from build123d import *
from build123d.topology import SkipClean

# Parameters (mm, degrees)
SKETCH_1_R          = 1.5
EXTRUDE_1_DEPTH     = 15
SKETCH_2_R          = 5
SKETCH_2_R_2        = 1.5
EXTRUDE_2_DEPTH     = 4
FILLET_1_R          = 1
SKETCH_3_R          = 1.5
CUT_EXTRUDE_1_DEPTH = 19
SKETCH_4_R          = 3.4
CUT_EXTRUDE_3_DEPTH = 19


with BuildPart() as part:
    # 草图1 → 凸台-拉伸1 (new body)
    with BuildSketch(Plane.XY):
        with BuildLine():
            Line((0, 0), (50, 0))
            Line((50, 0), (50, 8))
            Line((50, 8), (27.250210303, 19.465036796))
            ThreePointArc((27.250210303, 19.465036796), (25, 20), (22.749789697, 19.465036796))
            Line((22.749789697, 19.465036796), (0, 8))
            Line((0, 8), (0, 0))
        make_face()
        with Locations((25, 15)):
            Circle(SKETCH_1_R, mode=Mode.SUBTRACT)
    extrude(amount=EXTRUDE_1_DEPTH)

    # 草图2 → 凸台-拉伸2 (add)
    with BuildSketch(Plane.XY.offset(15)):
        with Locations(Location((25, 15, 0), (0, 0, 116.746382546))):
            Circle(SKETCH_2_R)
        with Locations((25, 15)):
            Circle(SKETCH_2_R_2, mode=Mode.SUBTRACT)
    extrude(amount=EXTRUDE_2_DEPTH)

    # 圆角1
    fillet_1_edges = [part.edges().sort_by_distance(p)[0] for p in [
        (27.250210303, 10.534963204, 19),
    ]]
    fillet(fillet_1_edges, radius=FILLET_1_R)

    # 草图3 → 切除-拉伸1 (cut)
    with SkipClean():  # the faces are left unmerged after this step: merging them gives an invalid solid
        with BuildSketch(Plane.XZ):
            with Locations(Location((5.25, 3, 0), (0, 0, 270))):
                Circle(SKETCH_3_R)
            with Locations(Location((44.75, 3, 0), (0, 0, 270))):
                Circle(SKETCH_3_R)
        extrude(amount=-CUT_EXTRUDE_1_DEPTH, mode=Mode.SUBTRACT)

    # 草图4 → 切除-拉伸3 (cut)
    with SkipClean():  # the faces are left unmerged after this step: merging them gives an invalid solid
        with BuildSketch(Plane(origin=(0, 8, 0), x_dir=(-1, 0, 0), z_dir=(0, -1, 0))):
            with Locations((-44.75, -3)):
                Circle(SKETCH_4_R)
            with Locations((-5.25, -3)):
                Circle(SKETCH_4_R)
        extrude(amount=-CUT_EXTRUDE_3_DEPTH, mode=Mode.SUBTRACT)


solid = part.part
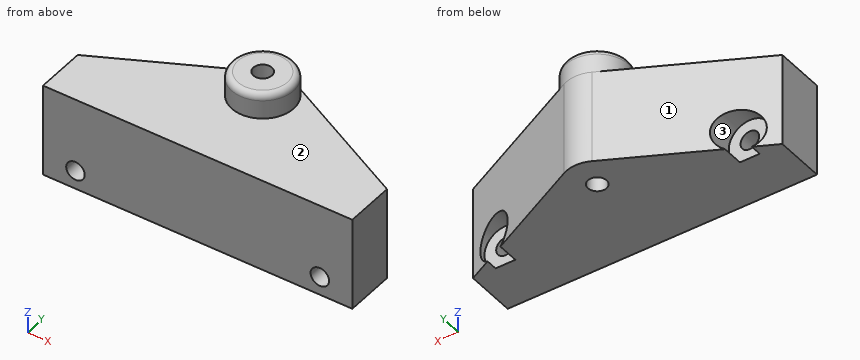
For this review, take the finished solid that the model builds, in its own axes (mm). Face numbers are marked on the shaded views. Round coordinates to 2 decimals unless told otherwise and drop trailing zeros. Write each loop counter-clockwise with the first axis right and the second up, starting at its lowest first coordinate (ties: lowest second). Pieces come first, ordered by that corner, then holes. Notation, with made-up numbers: (77, 87) -> (97, 87) arc R24 ccw to (97, 100) -> close; hole circle Ø2 at (24.25, 25.25). An arc over 180 degrees is marked (long way). Use CSV: the item, a comma, the result in double quotes.
(1) Consider section C-C, the plane y = 2.5. Give the boundary of the cut face in (x, z), plus the area to 3 significant figures.
Computed values:
outline,"(0, 0) -> (50, 0) -> (50, 15) -> (0, 15) -> close; hole circle Ø3 at (5.25, 3); hole circle Ø3 at (44.75, 3)"
area,"736 mm²"
(2) Consider section A-A, the plane z = 3. Give the boundary of the cut face in (x, y), plus the area to 3 significant figures.
Computed values:
outline,"(0, 0) -> (3.75, 0) -> (3.75, 8) -> (1.85, 8) -> (1.85, 8.93) -> (0, 8) -> close; (6.75, 0) -> (43.25, 0) -> (43.25, 8) -> (41.35, 8) -> (41.35, 12.36) -> (27.25, 19.47) arc R5 ccw to (22.75, 19.47) -> (8.65, 12.36) -> (8.65, 8) -> (6.75, 8) -> close; (46.25, 0) -> (50, 0) -> (50, 8) -> (48.15, 8.93) -> (48.15, 8) -> (46.25, 8) -> close; hole circle Ø3 at (25, 15)"
area,"623 mm²"
(3) Consider section D-D, the plane z = 14.5. Give the boundary of the cut face in (x, y).
Computed values:
outline,"(0, 0) -> (50, 0) -> (50, 8) -> (27.25, 19.47) arc R5 ccw to (22.75, 19.47) -> (0, 8) -> close; hole circle Ø3 at (25, 15)"
(4) Draft analysis for pull direction Z (two halves, no side actions). For the marked faces 1, 2 and 3, state which applies: +Z half, -Z half, draft (parallel to the pull), parting line (faces both ways), or undercut.
Computed values:
face 1,"draft"
face 2,"+Z half"
face 3,"undercut"
(5) Clearance check with flat-ended pins moving along their axes: P1, Ø6, axis at x = 44.75, z = 3, coming from the +Y side; P2, Ø6, axis at y = 17.5, z = 13.5, coming from the +X side; P3, Ø8, axis at x = 32.5, y = 3.5, coming from the +Z side. State where each tip first meets the part, or that it passes through.
Computed values:
P1,"y = 8"
P2,"x = 37.1"
P3,"z = 15"
(6) Consider section B-B, the plane x = 25. Give the boundary of the cut face in (y, z), plus the area to 3 significant figures.
Computed values:
outline,"(0, 0) -> (13.5, 0) -> (13.5, 19) -> (11, 19) arc R1 ccw to (10, 18) -> (10, 15) -> (0, 15) -> close; (16.5, 0) -> (20, 0) -> (20, 18) arc R1 ccw to (19, 19) -> (16.5, 19) -> close"
area,"283 mm²"
(7) To check wall thickness, follow L1, parallel to X at y = 4.5, z = 3; L2, parallel to Z at x = 41, y = 2; L3, parallel to Y at x = 25, z = 11. State the ranges of each line that lie inside material, in increasing order. Write a range as [from, to].
Computed values:
L1,"[0, 3.75], [6.75, 43.25], [46.25, 50]"
L2,"[0, 15]"
L3,"[0, 13.5], [16.5, 20]"
